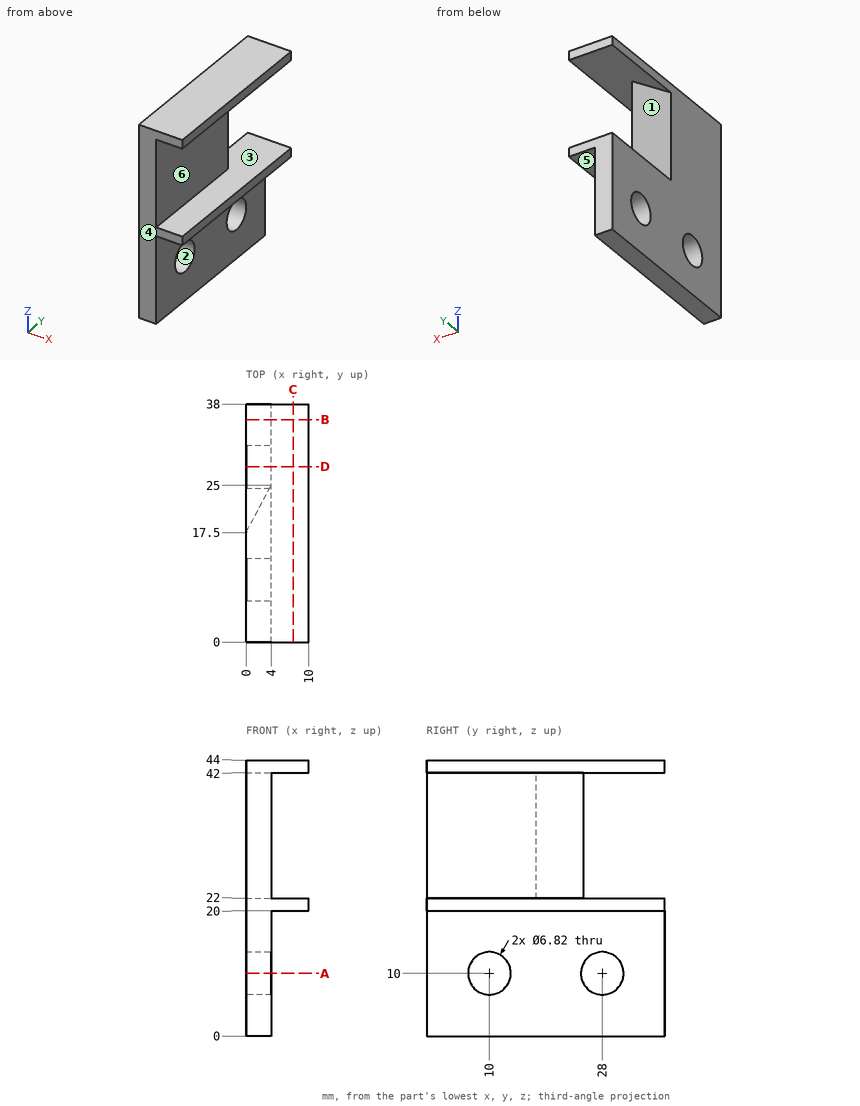
Verification items for this drawing (mm, ordinates from the low corner). A direction names the side the tool comes from. Round coordinates to 2 decimals unless told otherwise and drop trailing zeros. Write each loop counter-clockwise with the first axis right and the second up, starting at its lowest first coordinate (ties: lowest second). Pieces come first, ordered by that corner, then holes. Notation, with made-up numbers: (-20, 86) - (18, 86) arc R32 ccw to (18, 115) - close; hole circle Ø7 at (27, 72.25). An arc over 180 degrees is marked (long way). Answer as a JSON object with one key per item and string values. Group by question number.
Q1. Thickness scan on line 1 (Y direction, x = 2.45, z = 10); line 2 (Z direction, x = 6.75, y = 21.5); line 3 (Z direction, x = 2.5, y = 10.5). Record the ranges inside material, lowest first.
Q2. Mould release check, pull along Y, two halves, no side actions. Record for the marked faces 1, 2 and 3: released by +Y, released by -Y, zero draft, split by the parting line, or undercut.
Q3. Section check B-B, the plane y = 35.5. Enter the section's corners in (x, z), plus the area to 3 significant figures.
Q4. Section check A-A, the plane z = 10. Enter the section's corners in (x, y), plus the area to 3 significant figures.
Q5. Section check D-D, the plane y = 28. Enter the section's corners in (x, z), plus the area to 3 significant figures.
Q6. Go/stop test with flat-tipped pins: pin 1 Ø6 at (y, z) = (17.5, 10.5) entering from +X; pin 2 Ø1.8 at (x, y) = (7.5, 12) entering from -Z. Record where each tip stops, or that it passes through.
Q7. Section check C-C, the plane x = 7.5. Enter the section's corners in (y, z).
Q8. Tool access check on the marked faces 4, 5 and 6. Record the directions out of +Z, -Z, +X, -X, +Y, -Y that give a thin tool (end or side, any length) a straight path to the whole face; none if there is none.
Found:
{
 "1": {"line 1": "y = 0 to 6.59, 13.41 to 24.59, 31.41 to 38", "line 2": "z = 20 to 22, 42 to 44", "line 3": "z = 0 to 6.63, 13.37 to 44"},
 "2": {"face 1": "released by +Y", "face 2": "undercut", "face 3": "zero draft"},
 "3": {"outline": "(0, 0) - (4, 0) - (4, 20) - (10, 20) - (10, 22) - (0, 22) - close; (0, 42) - (10, 42) - (10, 44) - (0, 44) - close", "area": "120 mm^2"},
 "4": {"outline": "(0, 0) - (4, 0) - (4, 6.59) - (0, 6.59) - close; (0, 13.41) - (4, 13.41) - (4, 24.59) - (0, 24.59) - close; (0, 31.41) - (4, 31.41) - (4, 38) - (0, 38) - close", "area": "97.4 mm^2"},
 "5": {"outline": "(0, 0) - (4, 0) - (4, 6.59) - (0, 6.59) - close; (0, 13.41) - (4, 13.41) - (4, 20) - (10, 20) - (10, 22) - (0, 22) - close; (0, 42) - (10, 42) - (10, 44) - (0, 44) - close", "area": "92.7 mm^2"},
 "6": {"pin 1": "stops at x = 4", "pin 2": "stops at z = 20"},
 "7": {"outline": "(0, 20) - (38, 20) - (38, 22) - (0, 22) - close; (0, 42) - (38, 42) - (38, 44) - (0, 44) - close"},
 "8": {"face 4": "+Z, -Z, +X, -X, -Y", "face 5": "-Z, +X, +Y, -Y", "face 6": "+X, +Y, -Y"}
}
